Answer from the drawing. Dimensions are ordinates in mm from the lowest x, y and z of the part. A direction names the side the tool comes from. Round coordinates to 2 decimals unless told otherwise and drop trailing zeros. Loops run counter-clockwise (first coordinate to the right, second up) from the corner with the lowest first, then second, coordinate; pieces in that order, holes last. Notation, with made-up numbers: M -10,68 L 35,68 A13 cw 35,79 Z; hole C -26.75,66 d7. An arc over 180 degrees is marked long. Answer as CSV lines item,"result".
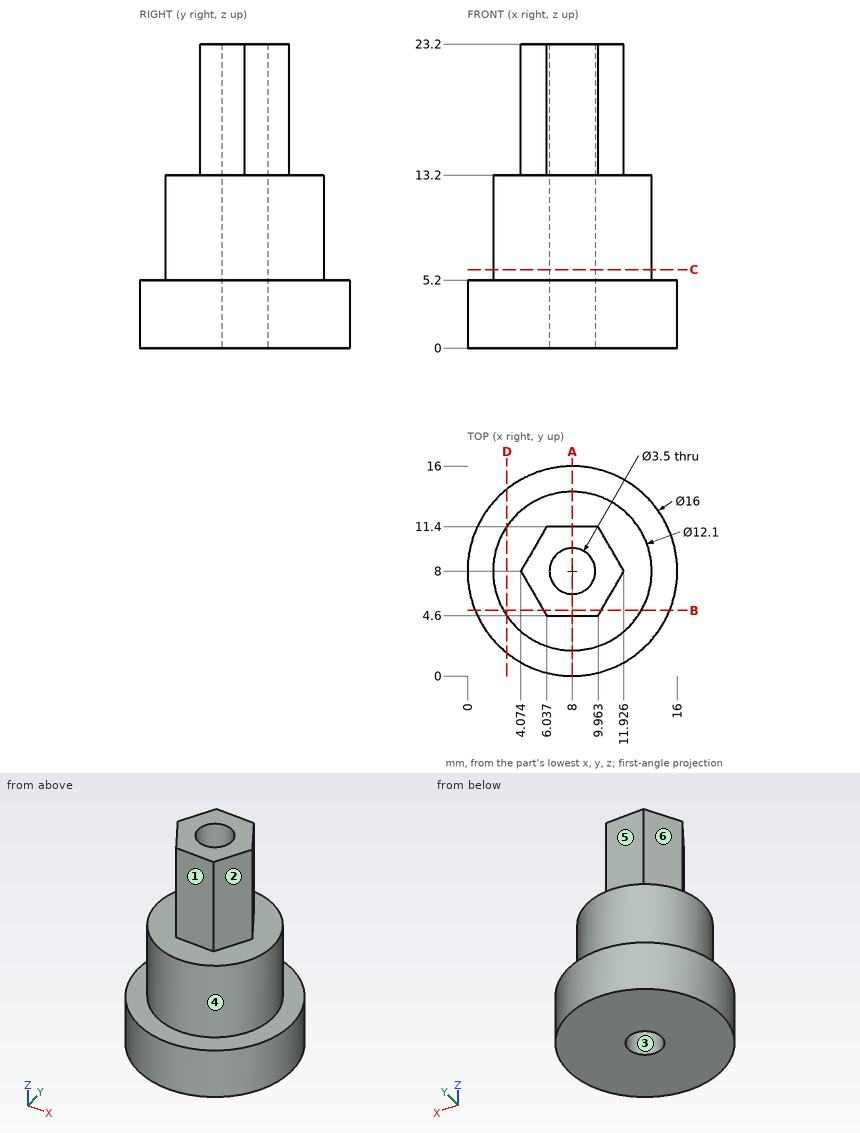
1) Find section B-B, the plane y = 5. Give the vertices of the cut face in (x, z).
Evaluation:
outline,"M 0.58,0 L 15.42,0 L 15.42,5.2 L 13.25,5.2 L 13.25,13.2 L 10.19,13.2 L 10.19,23.2 L 5.81,23.2 L 5.81,13.2 L 2.75,13.2 L 2.75,5.2 L 0.58,5.2 Z"
2) Find section C-C, the plane z = 6. Give the vertices of the cut face in (x, y), then the cut area to 3 significant figures.
Evaluation:
outline,"C 8,8 d12.1; hole C 8,8 d3.5"
area,"105 mm^2"
3) Determine the mould class of the marked faces 1, 2 and 3 for opening direction X: released by +X, released by -X, zero draft, split by the parting line, or undercut.
Evaluation:
face 1,"zero draft"
face 2,"released by +X"
face 3,"undercut"
4) A tool of negligible diameter and unlimited length cuts with its end or side. For the marked faces 4, 5 and 6, from which of +Z, -Z, +X, -X, +Y, -Y can it reach the whole face along a straight path? Write none if from no direction.
Evaluation:
face 4,"+Z"
face 5,"+Z, +X, -X, +Y"
face 6,"+Z, -X, +Y"
5) Each of these flat-tipped pins is pushed along its axis until it touches: P1, Ø1.2, axis at x = 7.5, z = 18.5, coming from the +Y side; P2, Ø8, axis at x = 2, z = 15, coming from the +Y side; P3, Ø1.2, axis at x = 8, z = 17, coming from the -Y side. Where does it stop, or does it pass through?
Evaluation:
P1,"stops at y = 11.4"
P2,"stops at y = 13.54"
P3,"stops at y = 4.6"
6) Find section D-D, the plane x = 3. Give the vertices of the cut face in (y, z) (3 decimals), then the cut area to 3 significant figures.
Evaluation:
outline,"M 1.755,0 L 14.245,0 L 14.245,5.2 L 11.406,5.2 L 11.406,13.2 L 4.594,13.2 L 4.594,5.2 L 1.755,5.2 Z"
area,"119 mm^2"
7) Straight lines are drawn through the part: line 1 (Y direction, x = 8, z = 10.25); line 2 (Y direction, x = 8, z = 16); line 3 (Z direction, x = 5.25, y = 12). For each, find the intervals that lie inside material, in ascending order.
Evaluation:
line 1,"y = 1.95 to 6.25, 9.75 to 14.05"
line 2,"y = 4.6 to 6.25, 9.75 to 11.4"
line 3,"z = 0 to 13.2"
8) Find section A-A, the plane x = 8. Give the vertices of the cut face in (y, z).
Evaluation:
outline,"M 0,0 L 6.25,0 L 6.25,23.2 L 4.6,23.2 L 4.6,13.2 L 1.95,13.2 L 1.95,5.2 L 0,5.2 Z; M 9.75,0 L 16,0 L 16,5.2 L 14.05,5.2 L 14.05,13.2 L 11.4,13.2 L 11.4,23.2 L 9.75,23.2 Z"
